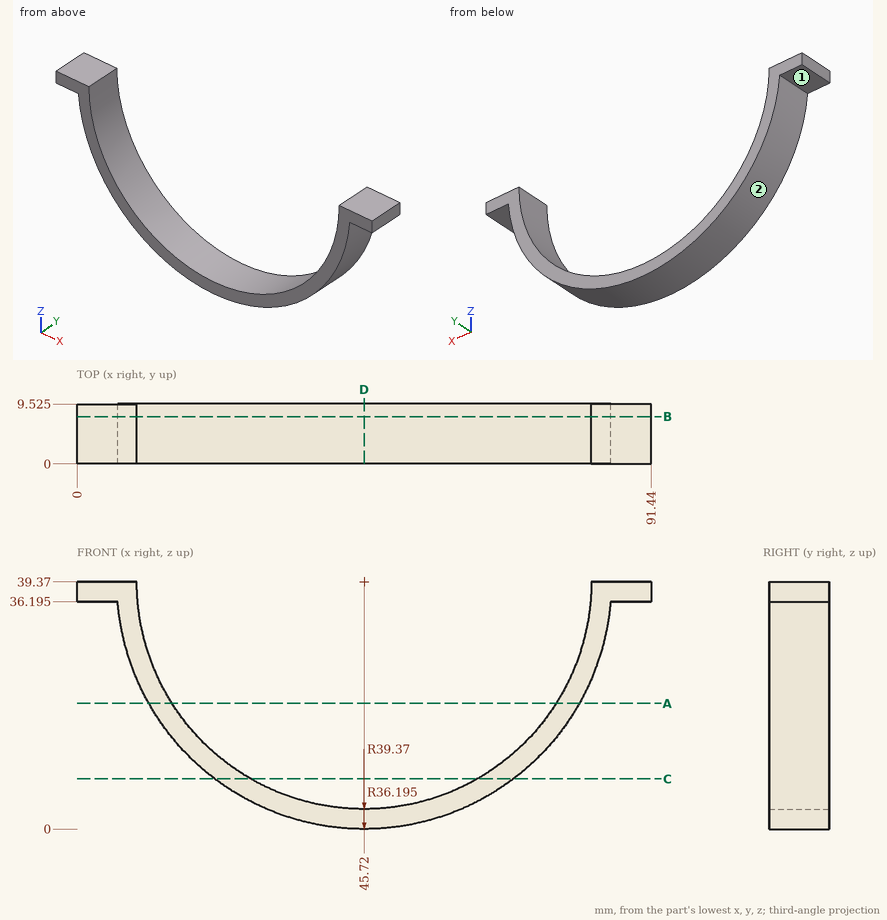
Design review of the part shown in the three views and the two pictorial views. Dimensions are in mm from the part's minimum x, y and z. A direction names the side the tool comes from. Give positions to 0.01 mm unless a question says otherwise; leave off trailing zeros. Loops run counter-clockwise (first coordinate to the right, second up) from the corner with the lowest first, then second, coordinate; pieces in that order, holes last. Notation, with made-up numbers: (76.25, 73.25) -> (126.25, 73.25) arc R17 cw to (126.25, 77.25) -> close; hole circle Ø3 at (62, 42.5). An arc over 180 degrees is marked (long way). Put each result on its own line as item: value. Start each with the question number.
1. Clearance check with flat-ended pins moving along their axes: P1, Ø1.5, axis at x = 11.5, y = 4.5, coming from the -Z side; P2, Ø3, axis at x = 72, z = 19, coming from the -Y side; P3, Ø5, axis at y = 6.5, z = 33.5, coming from the +X side; P4, Ø1.5, axis at x = 69.5, y = 3, coming from the -Z side. State where each tip first meets the part, or that it passes through.
2. We need section C-C on z = 8. State the section outline as (x, y) points (1 decimal), then the cut area to 3 significant figures.
3. We need section A-A on z = 20. State the section outline as (x, y) points (3 decimals).
4. We need section B-B on y = 7.5. State the section outline as (x, z) points (3 decimals), then the cut area to 3 significant figures.
5. We need section D-D on x = 45.72. State the section outline as (y, z) points (3 decimals).
6. Wall thickness on probe 1 along Z at (x, y) = (87.5, 9) (3 decimals); probe 2 along X at (y, z) = (3, 18.5); probe 3 along X at (y, z) = (5, 15): over which ranges is each line inside the solid? List them lowest first.
7. For the marked faces 1 and 2, list the 3-axis set-ups (+Z, -Z, +X, -X, +Y, -Y) from which the entire face can be reached by the end or side of a thin tool; tool diameter is ignored.
Determined:
1. P1: z = 18.64
1. P2: through
1. P3: x = 84.95
1. P4: z = 7.44
2. outline: (21.9, 0) -> (27.7, 0) -> (27.7, 9.5) -> (21.9, 9.5) -> close; (63.8, 0) -> (69.5, 0) -> (69.5, 9.5) -> (63.8, 9.5) -> close
2. area: 109 mm^2
3. outline: (11.445, 0) -> (15.144, 0) -> (15.144, 9.525) -> (11.445, 9.525) -> close; (76.296, 0) -> (79.995, 0) -> (79.995, 9.525) -> (76.296, 9.525) -> close
4. outline: (0, 36.195) -> (6.478, 36.195) arc R39.37 ccw to (84.962, 36.195) -> (91.44, 36.195) -> (91.44, 39.37) -> (81.915, 39.37) arc R36.195 cw to (9.525, 39.37) -> (0, 39.37) -> close
4. area: 417 mm^2
5. outline: (0, 0) -> (9.525, 0) -> (9.525, 3.175) -> (0, 3.175) -> close
6. probe 1: 36.195 to 39.37
6. probe 2: 12.34 to 16.15, 75.29 to 79.1
6. probe 3: 14.8 to 18.96, 72.48 to 76.64
7. face 1: -Z, -X, +Y, -Y
7. face 2: -Z, +Y, -Y
